Part model, mm, in its own coordinate system. Face numbers are marked on the shaded views. A direction names the side the tool comes from. Give positions to 0.01 mm unless a question says otherwise; leave off trailing zeros. Order: outer loops, then holes, each group sorted by start corner. A loop starts at its lowest first (then second) coordinate and runs counter-clockwise, first axis right, second up. Notation, with made-up numbers: (-20, 19.5) - (-6, 19.5) arc R32 ccw to (-6, 57.5) - close; hole circle Ø9 at (80, -26.5). An arc over 180 degrees is marked (long way). Use one line per item in the form item = value. Start each with the question number.
1. Pin check, flat tips, straight feed: P1, Ø1.5, axis at y = 3, z = 5, coming from the -X side; P2, Ø3, axis at y = -14.5, z = 2.5, coming from the +X side; P3, Ø2, axis at y = -24, z = 4.5, coming from the +X side. Stop position of each tip, or through.
2. Drill centre lines: line 1 (Y direction, x = 3, z = 2.75); line 2 (X direction, y = -21.5, z = -0.25); line 3 (Y direction, x = -1, z = -0.5). Where is each one in solid material? Low to high.
3. Band-saw the part on A-A, the plane x = 0. List the corners of the cut face in (y, z).
4. Tool access for the marked faces 1, 2 and 3: list every direction of +Z, -Z, +X, -X, +Y, -Y with a clear straight run to the whole face (end or side of a thin tool).
5. Band-saw the part on B-B, the plane y = 2.5. List the corners of the cut face in (x, z).
6. Pull direction Z, two halves, no side cores. Call the marked faces 4, 5, 6 and 7: +Z half, -Z half, draft (parallel to the pull), parting line (faces both ways), or undercut.
7. Band-saw the part on C-C, the plane y = -3. List the corners of the cut face in (x, z).
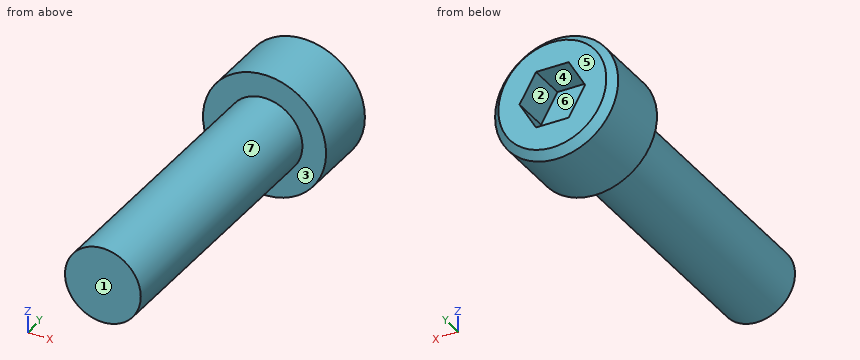
from build123d import *

# Parameters (mm, degrees)
CUT_EXTRUDE1_DEPTH = 4
CHAMFER1_SIZE      = 0.8


with BuildPart() as part:
    # Sketch1 → Revolve1 (revolve)
    with BuildSketch(Plane.XY):
        Polygon((0, 8), (6.5, 8), (6.5, 0), (4, 0), (4, -30), (0, -30), align=None)
    revolve(axis=Axis((0, 0, 0), (0, 1, 0)))

    # Sketch2 → Cut-Extrude1 (cut)
    with BuildSketch(Plane(origin=(0, 8, 0), x_dir=(1, 0, 0), z_dir=(0, 1, 0))):
        Polygon((3.464101615, 0), (1.732050808, 3), (-1.732050808, 3), (-3.464101615, 0), (-1.732050808, -3), (1.732050808, -3), align=None)
    extrude(amount=-CUT_EXTRUDE1_DEPTH, mode=Mode.SUBTRACT)

    # Chamfer1
    chamfer1_edges = [part.edges().sort_by_distance(p)[0] for p in [
        (-6.5, 8, 0),
    ]]
    chamfer(chamfer1_edges, length=CHAMFER1_SIZE)


solid = part.part
From the geometry:
q1.P1 = -4.92
q1.P2 = 3.87
q1.P3 = 1.94
q2.line_1 = 0 to 8
q2.line_2 = -3.99 to 3.99
q2.line_3 = -30 to 4
q3.outline = (-30, -4) - (0, -4) - (0, -6.5) - (7.2, -6.5) - (8, -5.7) - (8, -3) - (4, -3) - (4, 3) - (8, 3) - (8, 5.7) - (7.2, 6.5) - (0, 6.5) - (0, 4) - (-30, 4) - close
q4.face_1 = +Z, -Z, +X, -X, -Y
q4.face_2 = +Y
q4.face_3 = -Y
q5.outline = circle Ø13 at (0, 0)
q6.face_4 = undercut
q6.face_5 = draft
q6.face_6 = undercut
q6.face_7 = parting line
q7.outline = circle Ø8 at (0, 0)
